Here's how the part is built. I have some questions about the finished solid (model axes, mm). A direction names the side the tool comes from. Give positions to 0.01 mm unless a question says otherwise; leave off trailing zeros. Write each loop counter-clockwise with the first axis right and the second up, starting at its lowest first coordinate (ties: lowest second). Pieces come first, ordered by that corner, then holes. Notation, with made-up numbers: (45.5, 10.5) - (92.5, 10.5) arc R28 ccw to (92.5, 46.5) - close; hole circle Ø1 at (52, -27.75). An arc over 180 degrees is marked (long way). One line per item, written item: value. Start each with the question number.
1) Please list where these lines run through material, in increasing order: L1, parallel to X at y = 53.5, z = 193.5; L2, parallel to Z at x = 138, y = 161. Write a range as [from, to].
2) We'd pull the mould along X, two halves only. Please class faces 1 (the flat face through (0, 155, 100)), 2 (the flat face through (150, 0, 100)), 3 (the flat face through (151, 154, 25.4)): +X half, -X half, draft (parallel to the pull), parting line (faces both ways), or undercut.
3) Imagine slicing it at A-A on z = 56. Write out the boundary of the cut face in (x, y), plus the area to 3 significant figures.
4) I'm going to push flat-ended pins straight in: P1, Ø1.5, axis at x = 69.5, y = 63.5, coming from the +Z side; P2, Ø6, axis at x = 34, z = 135.5, coming from the -Y side. Where does each tip first touch, or does it pass through?
5) Imagine slicing it at B-B on y = 181.5. Write out the boundary of the cut face in (x, z).
6) On a 3-axis mill with a long thin cutter (end or side, diameter ignored), from which of +Z, -Z, +X, -X, +Y, -Y can I reach the whole of each face in a straight line? I mean faces 4 (the flat face through (25.4, 154, 113)), 5 (the flat face through (304.8, 150, 100)). Say none if no direction works.
Autodesk Inventor part; units mm, degrees
ref_plane "YZ Plane" through (0, 0, 0) normal (1, 0, 0) x (0, 1, 0)
ref_plane "XZ Plane" through (0, 0, 0) normal (0, 1, 0) x (-1, 0, 0)
ref_plane "XY Plane" through (0, 0, 0) normal (0, 0, 1) x (1, 0, 0)
sketch "Sketch1" plane through (0, 0, 0) normal (0, 0, 1) x (1, 0, 0)
  line L0 (0, 0) -> (304.8, 0)
  line L1 (304.8, 0) -> (304.8, 304.8)
  line L2 (304.8, 304.8) -> (0, 304.8)
  line L3 (0, 304.8) -> (0, 0)
  dimension "d0" = 304.8
  dimension "d1" = 304.8
extrude "Extrusion1" add sketch "Sketch1" along normal blind 203.2
shell "Shell1" thickness 25.4 removed faces 1 at (101.6, 203.2, 203.2)
equation "\"d1\" = d0"
properties part number "Yellow truck"
Numbers:
1. L1: [0, 25.4], [279.4, 304.8]
1. L2: [0, 25.4]
2. face 1: -X half
2. face 2: draft
2. face 3: undercut
3. outline: (0, 0) - (304.8, 0) - (304.8, 304.8) - (0, 304.8) - close; hole (25.4, 25.4) - (279.4, 25.4) - (279.4, 279.4) - (25.4, 279.4) - close
3. area: 28,400 mm^2
4. P1: z = 25.4
4. P2: y = 0
5. outline: (0, 0) - (304.8, 0) - (304.8, 203.2) - (279.4, 203.2) - (279.4, 25.4) - (25.4, 25.4) - (25.4, 203.2) - (0, 203.2) - close
6. face 4: +Z
6. face 5: +Z, -Z, +X, +Y, -Y
